```python
from build123d import *

# Parameters (mm, degrees)
CROQUIS1_R              = 27.5
SALIENTE_EXTRUIR1_DEPTH = 2.11
CROQUIS2_R              = 1.2
CROQUIS2_R_2            = 5
CROQUIS2_R_3            = 1.7
CORTAR_EXTRUIR1_DEPTH   = 3.11
REDONDEO1_R             = 2


with BuildPart() as part:
    # Croquis1 → Saliente-Extruir1 (new body)
    with BuildSketch(Plane(origin=(0, 0, 0), x_dir=(1, 0, 0), z_dir=(0, 1, 0))):
        Circle(CROQUIS1_R)
    extrude(amount=SALIENTE_EXTRUIR1_DEPTH)

    # Croquis2 → Cortar-Extruir1 (cut, through all)
    with BuildSketch(Plane(origin=(0, 2.11, 0), x_dir=(1, 0, 0), z_dir=(0, 1, 0))):
        with Locations((0, 15)):
            Circle(CROQUIS2_R)
        with Locations((12.990381057, -7.5)):
            Circle(CROQUIS2_R)
        with Locations((-12.990381057, -7.5)):
            Circle(CROQUIS2_R)
        Circle(CROQUIS2_R_2)
        with Locations((-14.722431864, 8.5)):
            Circle(CROQUIS2_R_3)
        with Locations((14.722431864, 8.5)):
            Circle(CROQUIS2_R_3)
        with Locations((0, -17)):
            Circle(CROQUIS2_R_3)
        with BuildLine():
            Line((-2.5, 6.538348415), (-2.5, 24.372115214))
            ThreePointArc((-2.5, 24.372115214), (-9.267968283, 22.679390731), (-15.28445201, 19.147729023))
            Line((-15.28445201, 19.147729023), (-11.324842647, 9.965055464))
            ThreePointArc((-11.324842647, 9.965055464), (-11.51813787, 6.65), (-14.292412506, 4.825073694))
            Line((-14.292412506, 4.825073694), (-24.224645764, 3.662859212))
            ThreePointArc((-24.224645764, 3.662859212), (-24.274912656, -3.313399391), (-22.356870919, -10.020994097))
            Line((-22.356870919, -10.020994097), (-6.912375826, -1.104110698))
            ThreePointArc((-6.912375826, -1.104110698), (-6.062177826, 3.5), (-2.5, 6.538348415))
        make_face()
        with BuildLine():
            Line((2.5, 6.538348415), (2.5, 24.372115214))
            ThreePointArc((2.5, 24.372115214), (9.267968283, 22.679390731), (15.28445201, 19.147729023))
            Line((15.28445201, 19.147729023), (11.324842647, 9.965055464))
            ThreePointArc((11.324842647, 9.965055464), (11.51813787, 6.65), (14.292412506, 4.825073694))
            Line((14.292412506, 4.825073694), (24.224645764, 3.662859212))
            ThreePointArc((24.224645764, 3.662859212), (24.274912656, -3.313399391), (22.356870919, -10.020994097))
            Line((22.356870919, -10.020994097), (6.912375826, -1.104110698))
            ThreePointArc((6.912375826, -1.104110698), (6.062177826, 3.5), (2.5, 6.538348415))
        make_face()
        with BuildLine():
            Line((4.412375826, -5.434237717), (19.856870919, -14.351121116))
            ThreePointArc((19.856870919, -14.351121116), (15.006944374, -19.36599134), (8.940193754, -22.810588235))
            Line((8.940193754, -22.810588235), (2.967569858, -14.790129159))
            ThreePointArc((2.967569858, -14.790129159), (0, -13.3), (-2.967569858, -14.790129159))
            Line((-2.967569858, -14.790129159), (-8.940193754, -22.810588235))
            ThreePointArc((-8.940193754, -22.810588235), (-15.006944374, -19.36599134), (-19.856870919, -14.351121116))
            Line((-19.856870919, -14.351121116), (-4.412375826, -5.434237717))
            ThreePointArc((-4.412375826, -5.434237717), (0, -7), (4.412375826, -5.434237717))
        make_face()
    extrude(amount=-CORTAR_EXTRUIR1_DEPTH, mode=Mode.SUBTRACT)

    # Redondeo1
    redondeo1_edges = [part.edges().sort_by_distance(p)[0] for p in [
        (6.912375826, 1.055, 1.104110698),
        (2.5, 1.055, -6.538348415),
        (2.5, 1.055, -24.372115214),
        (15.28445201, 1.055, -19.147729023),
        (24.224645764, 1.055, -3.662859212),
        (22.356870919, 1.055, 10.020994097),
        (-4.412375826, 1.055, 5.434237717),
        (4.412375826, 1.055, 5.434237717),
        (19.856870919, 1.055, 14.351121116),
        (8.940193754, 1.055, 22.810588235),
        (-8.940193754, 1.055, 22.810588235),
        (-19.856870919, 1.055, 14.351121116),
        (-2.5, 1.055, -6.538348415),
        (-6.912375826, 1.055, 1.104110698),
        (-22.356870919, 1.055, 10.020994097),
        (-24.224645764, 1.055, -3.662859212),
        (-15.28445201, 1.055, -19.147729023),
        (-2.5, 1.055, -24.372115214),
    ]]
    fillet(redondeo1_edges, radius=REDONDEO1_R)


solid = part.part
```
Could you check a few things on this model? Use its own coordinates, in mm. Coordinates: 2 decimals unless noted, no trailing zeros. Order: outer loops, then holes, each group sorted by start corner. A loop starts at its lowest first (then second) coordinate and runs counter-clockwise, first axis right, second up. Notation, with made-up numbers: M 62.25,4.5 L 94.25,4.5 A25 ccw 94.25,17.5 Z; hole C -11,81.5 d9. An arc over 180 degrees is marked long. Use a Markdown table: item, result. Add a question column.
Q1. I want a section at B-B on z = 17. List the corners of the cut face in (x, y) for me.
Q2. I want a section at C-C on x = -21.5. List the corners of the cut face in (y, z) for me.
Q3. I want a section at D-D on z = -8.5. List the corners of the cut face in (x, y) for me.
Q4. I'm going to push flat-ended pins straight in: pin 1 (2.5 mm diameter, centred on x = 0, z = 17, fed in from +Y); pin 2 (1 mm diameter, centred on y = 1, z = -22, fed in from -X); pin 3 (1 mm diameter, centred on x = 17, y = 1.5, fed in from -Z). Where does each tip first touch, or does it pass through?
Q5. We'd pull the mould along Z, two halves only. Please class faces 1 (the cylindrical face through (-5.961, 1.04, 26.846)), 2 (the cylindrical face through (0, 1.1, 13.3)): pulls with the +Z half, pulls with the -Z half, needs draft (parallel to the pull), parting line crosses it, or undercut.
Q6. I want a section at A-A on x = 0. List the corners of the cut face in (y, z) for me.
Q7. If I drill on L1, parallel to Z at x = 0, y = 1.7; L2, parallel to X at y = 0.7, z = 0; L3, parallel to X at y = 0.95, z = -20, over which ranges is the centre line in solid material (lowest first)?
Checked values:
| question | item | result |
|---|---|---|
| 1 | outline | M -21.62,0 L -17.64,0 L -17.64,2.11 L -21.62,2.11 Z; M -4.61,0 L -1.7,0 L -1.7,2.11 L -4.61,2.11 Z; M 1.7,0 L 4.61,0 L 4.61,2.11 L 1.7,2.11 Z; M 17.64,0 L 21.62,0 L 21.62,2.11 L 17.64,2.11 Z |
| 2 | outline | M 0,-17.15 L 2.11,-17.15 L 2.11,-3.98 L 0,-3.98 Z; M 0,9.12 L 2.11,9.12 L 2.11,17.15 L 0,17.15 Z |
| 3 | outline | M -26.15,0 L -16.42,0 L -16.42,2.11 L -26.15,2.11 Z; M -13.02,0 L -11.02,0 L -11.02,2.11 L -13.02,2.11 Z; M -2.5,0 L 2.5,0 L 2.5,2.11 L -2.5,2.11 Z; M 11.02,0 L 13.02,0 L 13.02,2.11 L 11.02,2.11 Z; M 16.42,0 L 26.15,0 L 26.15,2.11 L 16.42,2.11 Z |
| 4 | pin 1 | through |
| 4 | pin 2 | x = -17.15 |
| 4 | pin 3 | z = -22 |
| 5 | face 1 | parting line crosses it |
| 5 | face 2 | undercut |
| 6 | outline | M 0,-27.5 L 2.11,-27.5 L 2.11,-16.2 L 0,-16.2 Z; M 0,-13.8 L 2.11,-13.8 L 2.11,-5 L 0,-5 Z; M 0,5 L 2.11,5 L 2.11,7 L 0,7 Z; M 0,13.3 L 2.11,13.3 L 2.11,15.3 L 0,15.3 Z; M 0,18.7 L 2.11,18.7 L 2.11,27.5 L 0,27.5 Z |
| 7 | L1 | -27.5 to -16.2, -13.8 to -5, 5 to 7, 13.3 to 15.3, 18.7 to 27.5 |
| 7 | L2 | -27.5 to -24.5, -7 to -5, 5 to 7, 24.5 to 27.5 |
| 7 | L3 | -18.87 to -14.13, -2.5 to 2.5, 14.13 to 18.87 |
